from build123d import *

# Parameters (mm, degrees)
SKETCH_1_W           = 40.2
SKETCH_1_H           = 30.2
SKETCH_1_W_2         = 20.2
SKETCH_1_H_2         = 20.2
EXTRUDE_1_DEPTH      = 50.8
EXTRUDE_2_DEPTH      = 10
EXTRUDE_2_DEPTH_BACK = 40.2
SKETCH_4_W           = 3.2
SKETCH_4_H           = 25.4
CUT_EXTRUDE_2_DEPTH  = 93.927513655
CHAMFER_1_SIZE       = 3.175
HOLE_WIZARD_M5_1_D   = 5.5
EXTRUDE_3_DEPTH      = 50.8
SKETCH_14_W          = 43.451610889
SKETCH_14_H          = 10
CUT_EXTRUDE_3_DEPTH  = 112.847190984


with BuildPart() as part:
    # Sketch 1 → Extrude 1 (new body)
    with BuildSketch(Plane.XY):
        with Locations((10.1, 10.1)):
            Rectangle(SKETCH_1_W, SKETCH_1_H)
        with Locations((10.1, 10.1)):
            Rectangle(SKETCH_1_W_2, SKETCH_1_H_2, mode=Mode.SUBTRACT)
    extrude(amount=EXTRUDE_1_DEPTH)

    # Sketch 3 → Extrude 2 (add, two sides: drawn at the far end of the back side and taken through both)
    with BuildSketch(Plane(origin=(0, 25.2, 0), x_dir=(1, 0, 0), z_dir=(0, 1, 0)).offset(-EXTRUDE_2_DEPTH_BACK)):
        with BuildLine():
            Line((-10, 0), (30.2, 0))
            add(Edge.make_bspline(
                [(30.2, 0), (36.683134474, 0.377878079), (55.880340128, 11.98777216), (58.933962636, 29.945985381), (59.393514037, 36.119152658)],
                knots=[0, 0, 0, 0, 0.46638288, 0.846265587, 0.846265587, 0.846265587, 0.846265587], degree=3))
            ThreePointArc((59.393514037, 36.119152658), (58.722687502, 37.138617507), (57.565727076, 36.75034004))
            ThreePointArc((57.565727076, 36.75034004), (10.1, 11.43), (-37.365727076, 36.75034004))
            ThreePointArc((-37.365727076, 36.75034004), (-38.522687502, 37.138617507), (-39.193514037, 36.119152658))
            add(Edge.make_bspline(
                [(-10, 0), (-16.483134474, 0.377878079), (-35.680340128, 11.98777216), (-38.733962636, 29.945985381), (-39.193514037, 36.119152658)],
                knots=[0, 0, 0, 0, 0.46638288, 0.846265587, 0.846265587, 0.846265587, 0.846265587], degree=3))
        make_face()
    extrude(amount=EXTRUDE_2_DEPTH + EXTRUDE_2_DEPTH_BACK)

    # Sketch 4 → Cut-Extrude 2 (cut, through all)
    with BuildSketch(Plane.ZY.offset(10)):
        with Locations((1.6, 10.1)):
            Rectangle(SKETCH_4_W, SKETCH_4_H)
    extrude(amount=-CUT_EXTRUDE_2_DEPTH, mode=Mode.SUBTRACT)

    # Chamfer 1
    chamfer_1_edges = [part.edges().sort_by_distance(p)[0] for p in [
        (0, 10.1, 50.8),
        (10.1, 0, 50.8),
        (20.2, 10.1, 50.8),
        (10.1, 20.2, 50.8),
    ]]
    chamfer(chamfer_1_edges, length=CHAMFER_1_SIZE)

    # Hole Wizard M5 _1 (through all)
    with Locations(Plane(origin=(30.2, 10.1, 38.1), x_dir=(0, 0, 1), z_dir=(1, 0, 0))):
        with Locations((0, 0), (-19.05, 0)):
            Hole(HOLE_WIZARD_M5_1_D / 2)

    # Sketch 12 → Extrude 3 (add)
    with BuildSketch(Plane.XY.offset(50.8)):
        with BuildLine():
            Line((-10, 25.2), (30.2, 25.2))
            ThreePointArc((30.2, 25.2), (10.1, 35.2), (-10, 25.2))
        make_face()
        with BuildLine():
            Line((-10, -5), (30.2, -5))
            ThreePointArc((30.2, -5), (10.1, -15), (-10, -5))
        make_face()
    extrude(amount=-EXTRUDE_3_DEPTH)

    # Sketch 14 → Cut-Extrude 3 (cut, through all)
    with BuildSketch(Plane.XY.offset(50.8)):
        with Locations((-31.725805445, 30.2)):
            Rectangle(SKETCH_14_W, SKETCH_14_H)
        with BuildLine():
            Line((10.1, 35.2), (-10, 35.2))
            Line((-10, 35.2), (-10, 25.2))
            ThreePointArc((-10, 25.2), (-1.125083519, 32.561917872), (10.1, 35.2))
        make_face()
        with Locations((-31.725805445, -10)):
            Rectangle(SKETCH_14_W, SKETCH_14_H)
        with BuildLine():
            ThreePointArc((30.2, -5), (21.325083519, -12.361917872), (10.1, -15))
            Line((10.1, -15), (30.2, -15))
            Line((30.2, -15), (73.651610889, -15))
            Line((73.651610889, -15), (73.651610889, -5))
            Line((73.651610889, -5), (30.2, -5))
        make_face()
        with BuildLine():
            Line((30.2, 35.2), (10.1, 35.2))
            ThreePointArc((10.1, 35.2), (21.325083519, 32.561917872), (30.2, 25.2))
            Line((30.2, 25.2), (73.651610889, 25.2))
            Line((73.651610889, 25.2), (73.651610889, 35.2))
            Line((73.651610889, 35.2), (30.2, 35.2))
        make_face()
        with BuildLine():
            ThreePointArc((10.1, -15), (-1.125083519, -12.361917872), (-10, -5))
            Line((-10, -5), (-10, -15))
            Line((-10, -15), (10.1, -15))
        make_face()
        with BuildLine():
            ThreePointArc((30.2, -5), (21.325083519, -12.361917872), (10.1, -15))
            Line((10.1, -15), (30.2, -15))
            Line((30.2, -15), (73.651610889, -15))
            Line((73.651610889, -15), (73.651610889, -5))
            Line((73.651610889, -5), (30.2, -5))
        make_face()
    extrude(amount=-CUT_EXTRUDE_3_DEPTH, mode=Mode.SUBTRACT)


solid = part.part
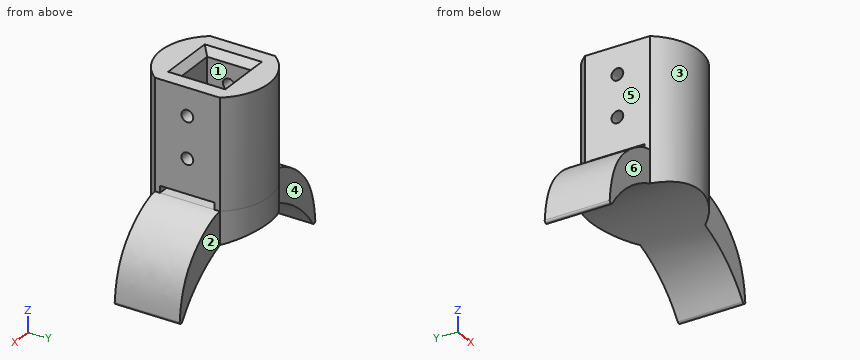
Verification items for the finished model (mm, model axes). Face numbers are marked on the shaded views. A direction names the side the tool comes from. Round coordinates to 2 decimals unless told otherwise and drop trailing zeros. Loops run counter-clockwise (first coordinate to the right, second up) from the corner with the lowest first, then second, coordinate; pieces in that order, holes last. Notation, with made-up numbers: M 33.25,36 L 56.25,36 A19 cw 56.25,70 Z; hole C 2.5,81.5 d10. An arc over 180 degrees is marked long. Write each question's results on one line, items separated by ' | '.
1) Section check B-B on y = 10.1. State how many separate pieces and enclosed holes the cut face has, then the cut area to 3 significant figures.
Checks:
separate pieces: 7 | enclosed holes: 0 | area: 2,120 mm2
2) Access from +Z, -Z, +X, -X, +Y, -Y to the whole of each face (thin tool, end or side, straight path). Record for the marked faces 4, 5 and 6.
Checks:
face 4: +Z, -Z, -X, +Y | face 5: +Z, -X, +Y, -Y | face 6: +Z, -Z, -X, -Y
3) Mould release check, pull along X, two halves, no side actions. Record for the marked faces 1, 2 and 3: released by +X, released by -X, zero draft, split by the parting line, or undercut.
Checks:
face 1: undercut | face 2: zero draft | face 3: split by the parting line
4) Gauge pin test, flat ends, axial feed: P1, Ø22, axis at y = 11.5, z = 32.5, coming from the +X side; P2, Ø2, axis at y = 7.5, z = 24, coming from the -X side; P3, Ø6, axis at x = 43.5, z = -15.5, coming from the +Y side. Record the tip position at first contact, or that the pin passes through.
Checks:
P1: stops at x = 30.2 | P2: stops at x = -10 | P3: stops at y = 25.2
5) Section check A-A on z = 38.1. Record the boundary of the cut face in (x, y).
Checks:
outline: M -10,-5 A25.2 ccw 30.2,-5 L 30.2,7.35 L 20.2,7.35 L 20.2,0 L 0,0 L 0,7.35 L -10,7.35 Z; M -10,12.85 L 0,12.85 L 0,20.2 L 20.2,20.2 L 20.2,12.85 L 30.2,12.85 L 30.2,25.2 A25.2 ccw -10,25.2 Z
6) Scan lines: L1, parallel to X at y = 12.5, z = 17; L2, parallel to Z at x = 27, y = 10.1; L3, parallel to Z at x = -2.5, y = 10.1 (3 decimals). Record each from-to range of solid material in increasing order. Write a range as from..to.
Checks:
L1: x = -10..0, 20.2..30.2 | L2: z = -13.99..0, 3.2..16.3, 21.8..35.35, 40.85..50.8 | L3: z = -12.836..0, 3.2..16.3, 21.8..35.35, 40.85..50.125
7) Section check C-C on x = 17. Record the boundary of the cut face in (y, z) (3 decimals).
Checks:
outline: M -14.037,-11.848 L 34.237,-11.848 L 34.237,50.8 L 23.375,50.8 L 20.2,47.625 L 20.2,3.2 L 22.8,3.2 L 22.8,0 L -2.6,0 L -2.6,3.2 L 0,3.2 L 0,47.625 L -3.175,50.8 L -14.037,50.8 Z
